Check sheet for the modelled part. Datum: model origin and axes. Units: mm. Face numbers are marked on the shaded views. A direction names the side the tool comes from. Round coordinates to 2 decimals unless told otherwise and drop trailing zeros. Loops run counter-clockwise (first coordinate to the right, second up) from the corner with the lowest first, then second, coordinate; pieces in that order, holes last. Notation, with made-up numbers: (8, 3) - (18, 3) arc R33 ccw to (18, 40) - close; hole circle Ø6 at (55.25, -38). An arc over 180 degrees is marked (long way). Put each result on its own line as item: value. Start each with the question number.
Item 1: Draft check along Z on the marked faces 4, 5 and 6. Enter one of: pulls with the +Z half, pulls with the -Z half, needs draft (parallel to the pull), parting line crosses it, or undercut.
Item 2: Section check B-B, the plane y = 4. Record the cut outline in (x, z), and give its area (3 significant figures).
Item 3: Tool access check on the marked faces 1, 2 and 3. Record the directions out of +Z, -Z, +X, -X, +Y, -Y that give a thin tool (end or side, any length) a straight path to the whole face; none if there is none.
Item 4: Gauge pin test, flat ends, axial feed: pin 1 Ø11 at (y, z) = (17.5, 15) entering from +X; pin 2 Ø9 at (x, z) = (17, 15) entering from +Y; pin 3 Ø10 at (x, y) = (25, 6.5) entering from +Z. Record the tip position at first contact, or that the pin passes through.
Item 5: Section check A-A, the plane z = 15. Record the cut outline in (x, y).
Item 6: Material ranges on line 1 along Z through (x, y) = (17.5, 1.35); line 2 along Z through (x, y) = (17.5, 3.05); line 3 along Y through (x, z) = (4.5, 14.75), recorded low to high.
Item 7: Section check D-D, the plane y = 18. Record the cut outline in (x, z).
Item 8: Section check C-C, the plane x = 26. Record the cut outline in (y, z).
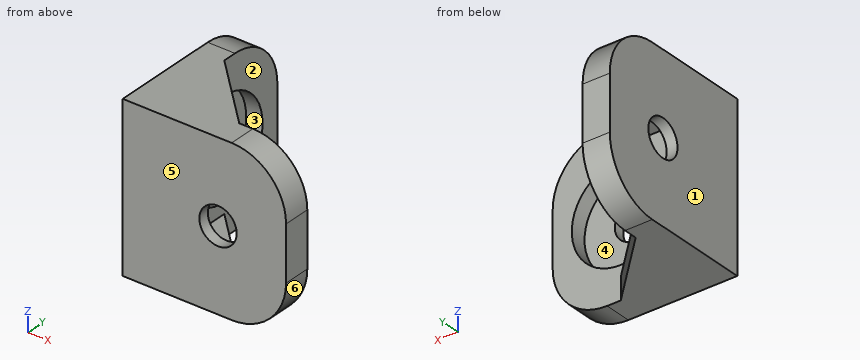
from build123d import *

# Parameters (mm, degrees)
BOSS_EXTRUDE1_DEPTH     = 30
SKETCH2_R               = 3.429
CUT_EXTRUDE1_DEPTH      = 50.244289009
CUT_EXTRUDE2_DEPTH      = 50.244289009
CUT_EXTRUDE2_DEPTH_BACK = 50.244289009
SKETCH4_R               = 3.429
SKETCH7_R               = 9
CUT_EXTRUDE3_DEPTH      = 3
SKETCH8_R               = 9
CUT_EXTRUDE4_DEPTH      = 3
BOSS_EXTRUDE2_DEPTH     = 4
BOSS_EXTRUDE3_DEPTH     = 4
FILLET1_R               = 10


with BuildPart() as part:
    # Sketch1 → Boss-Extrude1 (new body)
    with BuildSketch(Plane.XY):
        Polygon((0, 30), (0, 0), (30, 0), (30, 5), (5, 5), (5, 30), align=None)
    extrude(amount=BOSS_EXTRUDE1_DEPTH)

    # Sketch2 → Cut-Extrude1 (cut, through all)
    with BuildSketch(Plane(origin=(5, 0, 0), x_dir=(0, 0, -1), z_dir=(1, 0, 0))):
        with Locations(Location((-15, 17.5, 0), (0, 0, 90))):
            Circle(SKETCH2_R)
    extrude(amount=-CUT_EXTRUDE1_DEPTH, mode=Mode.SUBTRACT)

    # Sketch4 → Cut-Extrude2 (cut, two sides: drawn at the far end of the back side and taken through both)
    with BuildSketch(Plane(origin=(0, 5, 0), x_dir=(1, 0, 0), z_dir=(0, 1, 0)).offset(-CUT_EXTRUDE2_DEPTH_BACK)):
        with Locations(Location((17.5, -15, 0), (0, 0, 180))):
            Circle(SKETCH4_R)
    extrude(amount=CUT_EXTRUDE2_DEPTH + CUT_EXTRUDE2_DEPTH_BACK, mode=Mode.SUBTRACT)

    # Sketch7 → Cut-Extrude3 (cut)
    with BuildSketch(Plane(origin=(0, 5, 0), x_dir=(1, 0, 0), z_dir=(0, 1, 0))):
        with Locations(Location((17.5, -15, 0), (0, 0, 180))):
            Circle(SKETCH7_R)
    extrude(amount=-CUT_EXTRUDE3_DEPTH, mode=Mode.SUBTRACT)

    # Sketch8 → Cut-Extrude4 (cut)
    with BuildSketch(Plane(origin=(5, 0, 0), x_dir=(0, 0, -1), z_dir=(1, 0, 0))):
        with Locations(Location((-15, 17.5, 0), (0, 0, 90))):
            Circle(SKETCH8_R)
    extrude(amount=-CUT_EXTRUDE4_DEPTH, mode=Mode.SUBTRACT)

    # Sketch9 → Boss-Extrude2 (add)
    with BuildSketch(Plane(origin=(0, 0, 0), x_dir=(-1, 0, 0), z_dir=(0, 0, -1))):
        Polygon((-17.5, 5), (-5, 17.5), (-5, 5), align=None)
    extrude(amount=-BOSS_EXTRUDE2_DEPTH)

    # Sketch10 → Boss-Extrude3 (add)
    with BuildSketch(Plane.XY.offset(30)):
        Polygon((5, 5), (17.5, 5), (5, 17.5), align=None)
    extrude(amount=-BOSS_EXTRUDE3_DEPTH)

    # Fillet1
    fillet1_edges = [part.edges().sort_by_distance(p)[0] for p in [
        (30, 2.5, 30),
        (2.5, 30, 30),
        (30, 2.5, 0),
        (2.5, 30, 0),
    ]]
    fillet(fillet1_edges, radius=FILLET1_R)


solid = part.part
Check result:
1. face 4: undercut
1. face 5: needs draft
1. face 6: pulls with the -Z half
2. outline: (0, 0) - (20, 0) arc R10 ccw to (30, 10) - (30, 20) arc R10 ccw to (20, 30) - (0, 30) - close; hole circle Ø18 at (17.5, 15)
2. area: 603 mm²
3. face 1: +Z, -Z, -X, +Y, -Y
3. face 2: +X, +Y
3. face 3: +X
4. pin 1: x = 2
4. pin 2: y = 2
4. pin 3: z = 30
5. outline: (0, 0) - (14.07, 0) - (14.07, 2) - (8.5, 2) - (8.5, 5) - (5, 5) - (5, 8.5) - (2, 8.5) - (2, 14.07) - (0, 14.07) - close; (0, 20.93) - (2, 20.93) - (2, 26.5) - (5, 26.5) - (5, 30) - (0, 30) - close; (20.93, 0) - (30, 0) - (30, 5) - (26.5, 5) - (26.5, 2) - (20.93, 2) - close
6. line 1: 0 to 11.57, 18.43 to 30
6. line 2: 0 to 6, 24 to 30
6. line 3: 0 to 8.5, 26.5 to 30
7. outline: (0, 0) - (5, 0) - (5, 6.01) - (2, 6.01) - (2, 11.61) - (0, 11.61) - close; (0, 18.39) - (2, 18.39) - (2, 23.99) - (5, 23.99) - (5, 30) - (0, 30) - close
8. outline: (0, 2) - (5, 2) - (5, 12.04) - (2, 12.04) - (2, 17.96) - (5, 17.96) - (5, 28) - (0, 28) - close
